from build123d import *

# Parameters (mm, degrees)
SKETCH_W     = 90
SKETCH_H     = 65
SKETCH_R     = 1.5
PAD_DEPTH    = 3
PAD001_DEPTH = 7.3
PAD002_DEPTH = 15
FILLET_R     = 4
FILLET002_R  = 1
CHAMFER_SIZE = 2


with BuildPart() as part:
    # Sketch → Pad (new body)
    with BuildSketch(Plane.XY):
        with Locations((45, 32.5)):
            Rectangle(SKETCH_W, SKETCH_H)
        with Locations((27, 57)):
            Circle(SKETCH_R, mode=Mode.SUBTRACT)
        with Locations((85, 57)):
            Circle(SKETCH_R, mode=Mode.SUBTRACT)
        with Locations((85, 8)):
            Circle(SKETCH_R, mode=Mode.SUBTRACT)
        with Locations((27, 8)):
            Circle(SKETCH_R, mode=Mode.SUBTRACT)
    extrude(amount=PAD_DEPTH)

    # Sketch002 → Pad001 (join)
    with BuildSketch(Plane.XY):
        Polygon((85, 65), (85, 74), (84, 74), (84, 76), (85, 76), (85, 79), (72, 79), (72, 76), (73, 76), (73, 74), (72, 74), (72, 65), align=None)
    extrude(amount=PAD001_DEPTH)

    # Sketch003 → Pad002 (join)
    with BuildSketch(Plane.XY):
        with BuildLine():
            Line((25.5, 0), (25.5, -17))
            Line((25.5, -17), (32, -17))
            Line((32, -17), (32, -14))
            Line((32, -14), (29.5, -14))
            Line((29.5, -14), (29.5, -12.8))
            Line((29.5, -12.8), (34, -12.8))
            Line((34, -12.8), (34, -4.8))
            Line((34, -4.8), (59, -4.8))
            Line((59, -4.8), (59, -12.8))
            Line((59, -12.8), (61.825962, -12.8))
            ThreePointArc((61.825962, -12.8), (63.447393, -8.216284), (63.728416, -3.362367))
            ThreePointArc((65.223221, -3.237633), (64.413451, -2.552598), (63.728416, -3.362367))
            ThreePointArc((63.5, -12.8), (64.990453, -8.132139), (65.223221, -3.237633))
            Line((64.5, -12.8), (63.5, -12.8))
            Line((64.5, -14), (64.5, -12.8))
            Line((62.5, -14), (64.5, -14))
            Line((64.232051, -17), (62.5, -14))
            Line((71, -17), (64.232051, -17))
            Line((71, -11), (71, -17))
            Line((69, -11), (71, -11))
            Line((69, -14), (69, -11))
            Line((67, -14), (69, -14))
            Line((67, -14), (67, -12.8))
            ThreePointArc((69.968746, -3.3), (67.759472, -7.823469), (67, -12.8))
            ThreePointArc((69.968746, -3.3), (70.736182, -1.728691), (71, 0))
            Line((25.5, 0), (71, 0))
        make_face()
    extrude(amount=PAD002_DEPTH)

    # Fillet
    fillet_edges = [part.edges().sort_by_distance(p)[0] for p in [
        (90, 0, 1.5),
        (90, 65, 1.5),
        (0, 65, 1.5),
        (0, 0, 1.5),
    ]]
    fillet(fillet_edges, radius=FILLET_R)

    # Fillet002
    fillet002_edges = [part.edges().sort_by_distance(p)[0] for p in [
        (85, 79, 3.65),
        (72, 79, 3.65),
    ]]
    fillet(fillet002_edges, radius=FILLET002_R)

    # Chamfer
    chamfer_edges = [part.edges().sort_by_distance(p)[0] for p in [
        (78.5, 65, 3),
        (48.25, 0, 3),
    ]]
    chamfer(chamfer_edges, length=CHAMFER_SIZE)


solid = part.part
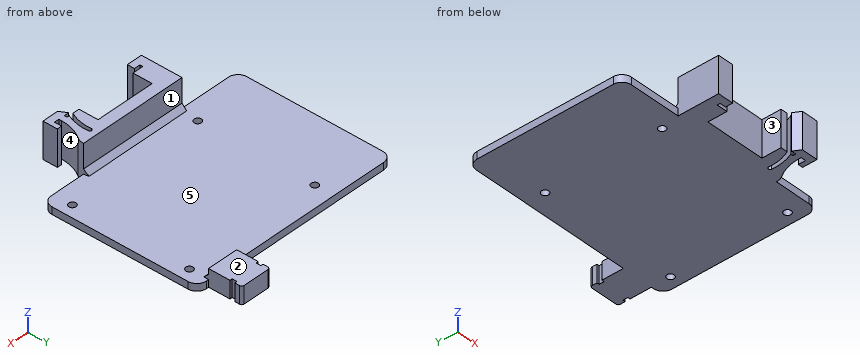
CAD build for the part. Positions are in the model's coordinates, mm. Face numbers are marked on the shaded views. A direction names the side the tool comes from. Coordinates: 2 decimals unless noted, no trailing zeros. Loops run counter-clockwise (first coordinate to the right, second up) from the corner with the lowest first, then second, coordinate; pieces in that order, holes last. Notation, with made-up numbers: (-18, 54) -> (11, 54) arc R31 cw to (11, 81) -> close; hole circle Ø9 at (39.25, -5.75). An arc over 180 degrees is marked (long way). One line per item, written item: value.
1. Slice it at B-B on y = 8. Write the cut outline in (x, z).
Answers:
outline: (0, 0) -> (25.5, 0) -> (25.5, 3) -> (0, 3) -> close; (28.5, 0) -> (83.5, 0) -> (83.5, 3) -> (28.5, 3) -> close; (86.5, 0) -> (90, 0) -> (90, 3) -> (86.5, 3) -> close
2. Slice it at A-A on x = 27. Write the cut outline in (y, z).
Answers:
outline: (-17, 0) -> (6.5, 0) -> (6.5, 3) -> (2, 3) -> (0, 5) -> (0, 15) -> (-17, 15) -> close; (9.5, 0) -> (55.5, 0) -> (55.5, 3) -> (9.5, 3) -> close; (58.5, 0) -> (65, 0) -> (65, 3) -> (58.5, 3) -> close
3. Drill centre lines: line 1 (Y direction, x = 27, z = 1.45); line 2 (Y direction, x = 85.5, z = 2.5); line 3 (X direction, y = -5, z = 14.75). Where is each one in solid material? Low to high. Write a range as [from, to].
Answers:
line 1: y = [-17, 6.5], [9.5, 55.5], [58.5, 65]
line 2: y = [0, 6.59], [9.41, 55.59], [58.41, 65]
line 3: x = [25.5, 34], [59, 63.79], [65.29, 68.94]
4. Which spindle directions (+Z, -Z, +X, -X, +Y, -Y) get a long thin tool onto all of the face, cutting with end or side? Do the marked faces 1, 2 and 3. Say none if no direction does.
Answers:
face 1: +Z, +X, -X, +Y
face 2: +Z, +X, -X, +Y, -Y
face 3: +Z, -Z, -Y
5. Slice it at D-D on z = 11.5. Write the cut outline in (x, y), and give its area (3 significant figures).
Answers:
outline: (25.5, -17) -> (32, -17) -> (32, -14) -> (29.5, -14) -> (29.5, -12.8) -> (34, -12.8) -> (34, -4.8) -> (59, -4.8) -> (59, -12.8) -> (61.83, -12.8) arc R17.29 ccw to (63.73, -3.36) arc R0.75 cw to (65.22, -3.24) arc R18.79 cw to (63.5, -12.8) -> (64.5, -12.8) -> (64.5, -14) -> (62.5, -14) -> (64.23, -17) -> (71, -17) -> (71, -11) -> (69, -11) -> (69, -14) -> (67, -14) -> (67, -12.8) arc R16.68 cw to (69.97, -3.3) arc R5.8 ccw to (71, 0) -> (25.5, 0) -> close
area: 393 mm^2
6. Pull direction X, two halves, no side cores. Call the marked faces 4 and 5: pulls with the +X half, pulls with the -X half, needs draft (parallel to the pull), parting line crosses it, or undercut.
Answers:
face 4: undercut
face 5: needs draft
7. Slice it at C-C on x = 60.5. Write the cut outline in (y, z), and give its area (3 significant figures).
Answers:
outline: (-12.8, 0) -> (65, 0) -> (65, 3) -> (2, 3) -> (0, 5) -> (0, 15) -> (-12.8, 15) -> close
area: 389 mm^2
8. Flat gauge pins, fed straight in: P1, Ø2.5, axis at y = -9.5, z = 5.5, coming from the -X side; P2, Ø3.5, axis at x = 85, y = 57, coming from the +Z side; P3, Ø0.8, axis at x = 72.5, z = 4.5, coming from the +Y side (3 decimals); P4, Ø1.8, axis at x = 85, y = 8, coming from the +Z side. Where does each tip first touch, or does it go through?
Answers:
P1: stops at x = 25.5
P2: stops at z = 3
P3: stops at y = 78.995
P4: passes through
